The drawing under review shows one solid part. Ordinate dimensions are in mm from its lowest x, y, z. A direction names the side the tool comes from. Coordinates: 2 decimals unless noted, no trailing zeros. Write each loop counter-clockwise with the first axis right and the second up, starting at its lowest first coordinate (ties: lowest second). Pieces come first, ordered by that corner, then holes.
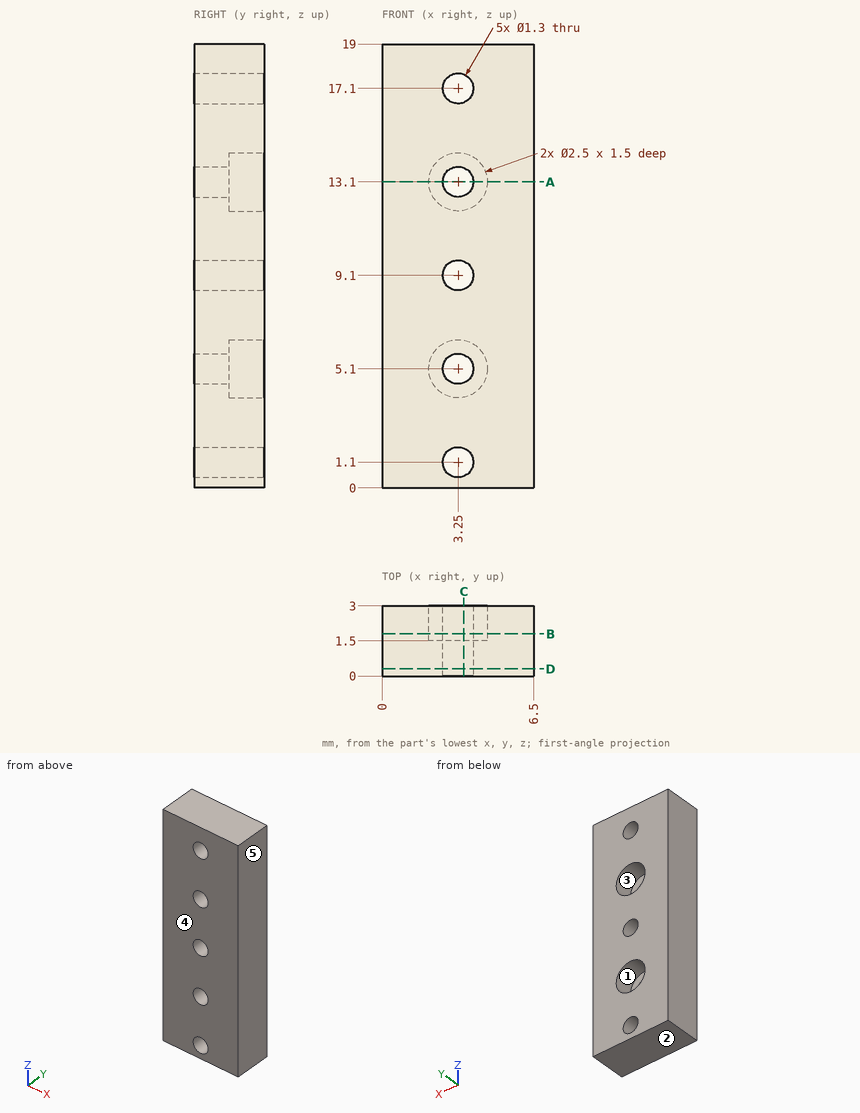
1) Clearance check with flat-ended pins moving along their axes: P1, Ø1, axis at x = 3.25, z = 13.1, coming from the +Y side (3 decimals); P2, Ø1.5, axis at x = 3.25, z = 13.1, coming from the +Y side. State where each tip first meets the part, or that it passes through.
2) The part is to be moulded in two halves that separate along X. For the marked faces 3, 4 and 5, say which applies: pulls with the +X half, pulls with the -X half, needs draft (parallel to the pull), parting line crosses it, or undercut.
3) For L1, parallel to Z at x = 3.25, y = 0.9; L2, parallel to Z at x = 3.25, y = 2; L3, parallel to X at y = 2.35, z = 13.1, list the stretches that pass through material, from the lowest coordinate up.
4) Consider section D-D (y = 0.3). Give the boundary of the cut face in (x, z).
5) Tool access review of the marked faces 1 and 2: name each direction out of +Z, -Z, +X, -X, +Y, -Y from which nothing blocks a thin tool from reaching the whole face with its end or side.
6) Consider section C-C (x = 3.5). Count the separate pieces of the cut face and the enclosed holes in it, then the cut area to 3 significant figures.
7) Consider section A-A (z = 13.1). Give the boundary of the cut face in (x, y).
8) Consider section B-B (y = 1.8). Give the boundary of the cut face in (x, z), then the cut area to 3 significant figures.
Results:
1. P1: passes through
1. P2: stops at y = 1.5
2. face 3: undercut
2. face 4: needs draft
2. face 5: pulls with the +X half
3. L1: z = 0 to 0.45, 1.75 to 4.45, 5.75 to 8.45, 9.75 to 12.45, 13.75 to 16.45, 17.75 to 19
3. L2: z = 0 to 0.45, 1.75 to 3.85, 6.35 to 8.45, 9.75 to 11.85, 14.35 to 16.45, 17.75 to 19
3. L3: x = 0 to 2, 4.5 to 6.5
4. outline: (0, 0) - (6.5, 0) - (6.5, 19) - (0, 19) - close; hole circle Ø1.3 at (3.25, 1.1); hole circle Ø1.3 at (3.25, 5.1); hole circle Ø1.3 at (3.25, 9.1); hole circle Ø1.3 at (3.25, 13.1); hole circle Ø1.3 at (3.25, 17.1)
5. face 1: +Y
5. face 2: -Z, +X, -X, +Y, -Y
6. separate pieces: 6
6. enclosed holes: 0
6. area: 35.3 mm2
7. outline: (0, 0) - (2.6, 0) - (2.6, 1.5) - (2, 1.5) - (2, 3) - (0, 3) - close; (3.9, 0) - (6.5, 0) - (6.5, 3) - (4.5, 3) - (4.5, 1.5) - (3.9, 1.5) - close
8. outline: (0, 0) - (6.5, 0) - (6.5, 19) - (0, 19) - close; hole circle Ø2.5 at (3.25, 5.1); hole circle Ø2.5 at (3.25, 13.1); hole circle Ø1.3 at (3.25, 1.1); hole circle Ø1.3 at (3.25, 9.1); hole circle Ø1.3 at (3.25, 17.1)
8. area: 110 mm2
